```python
from build123d import *

# Parameters (mm, degrees)
SKETCH2_R           = 9
BOSS_EXTRUDE1_DEPTH = 17
CUT_EXTRUDE1_DEPTH  = 4
SKETCH5_R           = 9
CUT_EXTRUDE3_DEPTH  = 11
SKETCH7_R           = 2.15
CUT_EXTRUDE4_DEPTH  = 7
SKETCH8_R           = 49
SKETCH8_R_2         = 1.3
BOSS_EXTRUDE2_DEPTH = 4
SKETCH9_W           = 6
SKETCH9_H           = 16
BOSS_EXTRUDE3_DEPTH = 13
FILLET1_R           = 3
SKETCH10_W          = 8
SKETCH10_H          = 5
CUT_EXTRUDE5_DEPTH  = 13


with BuildPart() as part:
    # Sketch2 → Boss-Extrude1 (new body)
    with BuildSketch(Plane.XY):
        with BuildLine():
            Line((14.881784229, -33.477238974), (14.881784229, -25.832605203))
            ThreePointArc((14.881784229, -25.832605203), (15.824526426, -20.598724896), (18.534251304, -16.022737899))
            ThreePointArc((18.534251304, -16.022737899), (15.896271469, 18.642831184), (-18.750548152, 15.769069256))
            Line((-18.750548152, 15.769069256), (-41.495728933, -15.659285702))
            ThreePointArc((-41.495728933, -15.659285702), (-44.193480097, -20.402788352), (-45.797718556, -25.618638973))
            Line((-45.797718556, -25.618638973), (-45.797718556, -33.477238974))
            Line((-45.797718556, -33.477238974), (14.881784229, -33.477238974))
        make_face()
        Circle(SKETCH2_R, mode=Mode.SUBTRACT)
    extrude(amount=BOSS_EXTRUDE1_DEPTH)

    # Sketch4 → Cut-Extrude1 (cut)
    with BuildSketch(Plane(origin=(0, 0, 0), x_dir=(-1, 0, 0), z_dir=(0, 0, -1))):
        with BuildLine():
            Line((-11.881784229, -30.477238974), (-11.881784229, -33.477238974))
            Line((-11.881784229, -33.477238974), (42.797718556, -33.477238974))
            Line((42.797718556, -33.477238974), (42.797718556, -30.477238974))
            Line((42.797718556, -30.477238974), (42.797718556, -25.912200391))
            ThreePointArc((42.797718556, -25.912200391), (41.384433584, -21.466180319), (39.065414716, -17.418141241))
            Line((39.065414716, -17.418141241), (16.386356383, 13.918848439))
            ThreePointArc((16.386356383, 13.918848439), (-13.989938582, 16.325704757), (-16.264744719, -14.060764438))
            ThreePointArc((-16.264744719, -14.060764438), (-13.013074866, -19.551948835), (-11.881784229, -25.832605203))
            Line((-11.881784229, -25.832605203), (-11.881784229, -30.477238974))
        make_face()
    extrude(amount=-CUT_EXTRUDE1_DEPTH, mode=Mode.SUBTRACT)

    # Sketch5 → Cut-Extrude3 (cut)
    with BuildSketch(Plane(origin=(0, 0, 4), x_dir=(-1, 0, 0), z_dir=(0, 0, -1))):
        Polygon((-14.849242405, 0.707106781), (-0.707106781, 14.849242405), (27.577164466, -13.435028843), (13.435028843, -27.577164466), align=None)
        Circle(SKETCH5_R, mode=Mode.SUBTRACT)
    extrude(amount=-CUT_EXTRUDE3_DEPTH, mode=Mode.SUBTRACT)

    # Sketch7 → Cut-Extrude4 (cut)
    with BuildSketch(Plane(origin=(0, 0, 4), x_dir=(-1, 0, 0), z_dir=(0, 0, -1))):
        with Locations((-6.590235201, 15.330075016)):
            Circle(SKETCH7_R)
        with Locations((-14.580541828, 7.339768389)):
            Circle(SKETCH7_R)
        with Locations(Location((20.06769045, -27.308463889, 0), (0, 0, 180))):
            Circle(SKETCH7_R)
        with Locations(Location((28.057997077, -19.318157262, 0), (0, 0, 180))):
            Circle(SKETCH7_R)
    extrude(amount=-CUT_EXTRUDE4_DEPTH, mode=Mode.SUBTRACT)

    # Sketch8 → Boss-Extrude2 (add)
    with BuildSketch(Plane.XZ.offset(33.477238974)):
        with Locations(Location((-11.457967164, 25, 0), (0, 0, 270))):
            Circle(SKETCH8_R)
        with Locations(Location((-18.807967164, 25, 0), (0, 0, 270))):
            Circle(SKETCH8_R_2, mode=Mode.SUBTRACT)
        with Locations(Location((-4.107967164, 25, 0), (0, 0, 270))):
            Circle(SKETCH8_R_2, mode=Mode.SUBTRACT)
    extrude(amount=BOSS_EXTRUDE2_DEPTH)

    # Sketch9 → Boss-Extrude3 (add)
    with BuildSketch(Plane(origin=(0, -33.477238974, 0), x_dir=(1, 0, 0), z_dir=(0, 1, 0))):
        with Locations((-31.797718556, -27)):
            Rectangle(SKETCH9_W, SKETCH9_H)
    extrude(amount=BOSS_EXTRUDE3_DEPTH)

    # Fillet1
    fillet1_edges = [part.edges().sort_by_distance(p)[0] for p in [
        (-31.797718556, -20.477238974, 35),
        (-31.797718556, -20.477238974, 19),
    ]]
    fillet(fillet1_edges, radius=FILLET1_R)

    # Sketch10 → Cut-Extrude5 (cut)
    with BuildSketch(Plane.ZY.offset(34.797718556)):
        with Locations((27, -26.977238974)):
            Rectangle(SKETCH10_W, SKETCH10_H)
    extrude(amount=-CUT_EXTRUDE5_DEPTH, mode=Mode.SUBTRACT)


solid = part.part
```
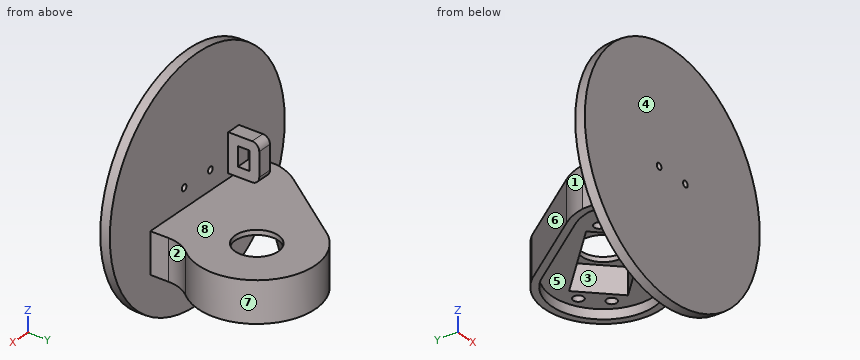
Input: part model. Units: mm. Frame: model coordinates. Face numbers are marked on the shaded views. A direction names the side the tool comes from. Give positions to 0.01 mm unless a question says otherwise; leave off trailing zeros. Order: outer loops, then holes, each group sorted by start corner. A loop starts at its lowest first (then second) coordinate and runs counter-clockwise, first axis right, second up. Notation, with made-up numbers: M 69.25,66 L 80.25,66 A27 cw 80.25,90 Z; hole C -8.75,36 d5. An arc over 180 degrees is marked long. Return JSON: item names as keys, results as strings.
Item 1: Pull-direction query (X, two-part tool) for the marked faces 5, 6, 7 and 8; classes: +X half, -X half, draft (parallel to the pull), parting line (faces both ways), or undercut.
Solutions:
{"face 5": "undercut", "face 6": "-X half", "face 7": "parting line", "face 8": "draft"}
Item 2: First-contact query: P1, Ø8, axis at x = -1, z = -9.5, coming from the +Y side; P2, Ø8, axis at y = -2.5, z = 13.5, coming from the +X side; P3, Ø5, axis at x = 6.59, y = 15.33, coming from the +Z side. Flat tips, straight axial feed; report the tip coordinate or a pass-through.
Solutions:
{"P1": "y = -33.48", "P2": "x = 24.5", "P3": "z = 17"}
Item 3: Access query for the marked faces 1, 2, 3 and 4. Directions: +Z, -Z, +X, -X, +Y, -Y. A direction counts if a zero-diameter tool reaches every point of the face in a straight line with its end or side. Return the directions, or none.
Solutions:
{"face 1": "+Z, -Z, -X, +Y", "face 2": "+Z, -Z, +X", "face 3": "-Z", "face 4": "+Z, -Z, +X, -X, -Y"}
Item 4: Cut plane A-A (z = 25). Return loops of the section in (x, y).
Solutions:
{"outline": "M -60.46,-37.48 L -20.11,-37.48 L -20.11,-33.48 L -28.8,-33.48 L -28.8,-29.48 L -34.8,-29.48 L -34.8,-33.48 L -60.46,-33.48 Z; M -34.8,-24.48 L -28.8,-24.48 L -28.8,-20.48 L -34.8,-20.48 Z; M -17.51,-37.48 L -5.41,-37.48 L -5.41,-33.48 L -17.51,-33.48 Z; M -2.81,-37.48 L 37.54,-37.48 L 37.54,-33.48 L -2.81,-33.48 Z"}
Item 5: Cut plane B-B (y = 2). Return loops of the section in (x, z).
Solutions:
{"outline": "M -28.72,0 L -25.01,0 L -25.01,4 L -12.14,4 L -12.14,15 L -8.77,15 L -8.77,17 L -28.72,17 Z; M 8.77,15 L 13.56,15 L 13.56,4 L 21.41,4 L 21.41,0 L 24.42,0 L 24.42,17 L 8.77,17 Z"}
Item 6: Ray query, probe 1 along X at (y, z) = (-36.1, 25); probe 2 along X at (y, z) = (9, 9.5); probe 3 along Y at (x, z) = (-10, 37). Return the intervals inside material, ascending.
Solutions:
{"probe 1": "-60.46 to -20.11, -17.51 to -5.41, -2.81 to 37.54", "probe 2": "-23.65 to -5.14, 6.56 to 13.21, 15.95 to 22.79", "probe 3": "-37.48 to -33.48"}
Item 7: Cut plane C-C (z = 8). Return loops of the section in (x, y), then the cut area to 3 significant figures.
Solutions:
{"outline": "M -57.41,-37.48 L 34.5,-37.48 L 34.5,-33.48 L 14.88,-33.48 L 14.88,-25.83 A15 cw 18.53,-16.02 A24.5 ccw long -18.75,15.77 L -41.5,-15.66 A25 ccw -45.8,-25.62 L -45.8,-33.48 L -57.41,-33.48 Z; hole C -28.06,-19.32 d4.3; hole M -27.58,-13.44 L -13.44,-27.58 L 14.85,0.71 L 0.71,14.85 Z; hole C -20.07,-27.31 d4.3; hole C 6.59,15.33 d4.3; hole C 14.58,7.34 d4.3", "area": "2,470 mm^2"}
Item 8: Cut plane D-D (z = -6.5). Return loops of the section in (x, y), then the cut area to 3 significant figures.
Solutions:
{"outline": "M -48.99,-37.48 L 26.08,-37.48 L 26.08,-33.48 L -48.99,-33.48 Z", "area": "300 mm^2"}
